Read the model definition and answer for the solid it produces. Units are mm, in the model's axes. Coordinates: 2 decimals unless noted, no trailing zeros. Loops run counter-clockwise (first coordinate to the right, second up) from the corner with the lowest first, then second, coordinate; pieces in that order, holes last. Notation, with made-up numbers: (17, 71.25) -> (59, 71.25) arc R21 ccw to (59, 77.25) -> close; hole circle Ø3 at (45.5, -1.5). An arc over 180 degrees is marked (long way). Answer as CSV lines item,"result".
```python
from build123d import *

# Parameters (mm, degrees)
EXTRUDE1_DEPTH     = 12.7
SKETCH3_R          = 3.1115
CUT_EXTRUDE1_DEPTH = 12.7


with BuildPart() as part:
    # Sketch2 → Extrude1 (new body)
    with BuildSketch(Plane.XY):
        with BuildLine():
            Line((10375.902142089, 13017.500110193), (10461.202782059, 13017.500110193))
            Line((10461.202782059, 13017.500110193), (10461.202782059, 13081.594724716))
            ThreePointArc((10461.202782059, 13081.594724716), (10463.062653998, 13086.084852777), (10467.552782059, 13087.944724716))
            Line((10467.552782059, 13087.944724716), (10554.77765388, 13087.944724716))
            ThreePointArc((10554.77765388, 13087.944724716), (10557.466824452, 13087.347190416), (10559.649893716, 13085.667043341))
            Line((10559.649893716, 13085.667043341), (10616.625223517, 13017.500110193))
            Line((10616.625223517, 13017.500110193), (10804.525747814, 13017.500110193))
            Line((10804.525747814, 13017.500110193), (10804.525747814, 13110.590509206))
            ThreePointArc((10804.525747814, 13110.590509206), (10798.175747814, 13116.940509206), (10804.525747814, 13123.290509206))
            Line((10804.525747814, 13123.290509206), (10852.150747814, 13123.290509206))
            Line((10852.150747814, 13123.290509206), (10852.147924282, 14185.900110193))
            Line((10852.147924282, 14185.900110193), (10337.800747814, 14185.900110193))
            Line((10337.800747814, 14185.900110193), (10337.802142089, 13109.003009206))
            Line((10337.802142089, 13109.003009206), (10369.552142089, 13109.003009206))
            ThreePointArc((10369.552142089, 13109.003009206), (10374.042270149, 13107.143137266), (10375.902142089, 13102.653009206))
            Line((10375.902142089, 13102.653009206), (10375.902142089, 13017.500110193))
        make_face()
    extrude(amount=-EXTRUDE1_DEPTH)

    # Sketch3 → Cut-Extrude1 (cut)
    with BuildSketch(Plane.XY):
        with Locations((10385.425050678, 13062.712110193)):
            Circle(SKETCH3_R)
        with Locations((10385.425050678, 13037.312110193)):
            Circle(SKETCH3_R)
        with Locations((10788.015050678, 13062.712110193)):
            Circle(SKETCH3_R)
        with Locations((10788.015050678, 13037.312110193)):
            Circle(SKETCH3_R)
    extrude(amount=-CUT_EXTRUDE1_DEPTH, mode=Mode.SUBTRACT)


solid = part.part
```
Q1. For a pull along X with two mould halves and no side action, classify faces 1 (the face through (10587.74, 13052.06, -6.26)), 2 (the face through (10591, 13610, 0)) as pulls with the +X half, pulls with the -X half, needs draft (parallel to the pull), parting line crosses it, or undercut.
Results:
face 1,"undercut"
face 2,"needs draft"
Q2. A cutting plane is placed at B-B, the plane x = 10490. Write down the section's boundary in (y, z), and give its area (3 significant figures).
Results:
outline,"(13087.94, -12.7) -> (14185.9, -12.7) -> (14185.9, 0) -> (13087.94, 0) -> close"
area,"13,900 mm²"
Q3. Given pin 1 Ø4 at (y, z) = (13052.5, -4) entering from +X; pin 2 Ø6.5 at (y, z) = (13072.5, -6.5) entering from -X; pin 3 Ø3 at (x, z) = (10525.5, -5.5) entering from -Y, each flat-ended and moving along its own axis, determine where each tip first touches the part or whether it passes through.
Results:
pin 1,"stops at x = 10804.53"
pin 2,"stops at x = 10375.9"
pin 3,"stops at y = 13087.94"
Q4. Find the intervals of material crossed by probe 1 along X at (y, z) = (13932.5, -7.5); probe 2 along Y at (x, z) = (10362.5, -5.5), in increasing order. Write a range as [from, to].
Results:
probe 1,"x = [10337.8, 10852.15]"
probe 2,"y = [13109, 14185.9]"
Q5. A cutting plane is placed at A-A, the plane z = -4.5. Write down the section's boundary in (x, y).
Results:
outline,"(10337.8, 13109) -> (10369.55, 13109) arc R6.35 cw to (10375.9, 13102.65) -> (10375.9, 13017.5) -> (10461.2, 13017.5) -> (10461.2, 13081.59) arc R6.35 cw to (10467.55, 13087.94) -> (10554.78, 13087.94) arc R6.35 cw to (10559.65, 13085.67) -> (10616.63, 13017.5) -> (10804.53, 13017.5) -> (10804.53, 13110.59) arc R6.35 cw to (10804.53, 13123.29) -> (10852.15, 13123.29) -> (10852.15, 14185.9) -> (10337.8, 14185.9) -> close; hole circle Ø6.22 at (10385.43, 13037.31); hole circle Ø6.22 at (10385.43, 13062.71); hole circle Ø6.22 at (10788.02, 13037.31); hole circle Ø6.22 at (10788.02, 13062.71)"
